For this review, take the finished solid that the model builds, in its own axes (mm). A direction names the side the tool comes from. Give positions to 0.01 mm unless a question says otherwise; leave off trailing zeros. Loops run counter-clockwise (first coordinate to the right, second up) from the corner with the lowest first, then second, coordinate; pieces in that order, holes last. Notation, with made-up numbers: (49, 3.25) - (94, 3.25) arc R24 ccw to (94, 33.25) - close; hole circle Ø5 at (39, 86.5). An arc over 180 degrees is marked (long way). Answer in a Markdown table with one row per item.
```python
from build123d import *

# Parameters (mm, degrees)
F0_W     = 160
F0_H     = 96
F0_W_2   = 143
F0_H_2   = 84
F0_R     = 1.5
F1_DEPTH = 10
F2_T     = -2


with BuildPart() as f1:
    # F0 (on Top) → F1 (new body)
    with BuildSketch(Plane.XY):
        Rectangle(F0_W, F0_H)
        Rectangle(F0_W_2, F0_H_2, mode=Mode.SUBTRACT)
        Rectangle(F0_W_2, F0_H_2)
        with Locations((-67.5, -38)):
            Circle(F0_R, mode=Mode.SUBTRACT)
        with Locations((67.5, -38)):
            Circle(F0_R, mode=Mode.SUBTRACT)
        with Locations((-67.5, 38)):
            Circle(F0_R, mode=Mode.SUBTRACT)
        with Locations((67.5, 38)):
            Circle(F0_R, mode=Mode.SUBTRACT)
    extrude(amount=F1_DEPTH)

    # F2
    f2_openings = [f1.faces().sort_by_distance(p)[0] for p in [
        (0, 0, 10),
    ]]
    offset(amount=F2_T, openings=f2_openings)


solid = f1.part
```
1. We need section D-D, the plane y = 15.5. Give the boundary of the cut face in (x, z).
Values:
| item | result |
|---|---|
| outline | (-80, 0) - (80, 0) - (80, 10) - (78, 10) - (78, 2) - (-78, 2) - (-78, 10) - (-80, 10) - close |
2. For faces 1 (the face through (68.886, -38.575, 4.93)), 2 (the face through (64.92, -35.635, 5.944)), list the 3-axis set-ups (+Z, -Z, +X, -X, +Y, -Y) from which the entire face can be reached by the end or side of a thin tool; tool diameter is ignored.
Values:
| item | result |
|---|---|
| face 1 | +Z, -Z |
| face 2 | +Z |
3. Wall thickness on line 1 (Y direction, x = 9, z = 7); line 2 (X direction, y = -34, z = 7.5); line 3 (Y direction, x = -67.5, z = 7.25): over which ranges is each line inside the solid? List them lowest first. Write a range as [from, to].
Values:
| item | result |
|---|---|
| line 1 | y = [-48, -46], [46, 48] |
| line 2 | x = [-80, -78], [78, 80] |
| line 3 | y = [-48, -46], [-41.5, -39.5], [-36.5, -34.5], [34.5, 36.5], [39.5, 41.5], [46, 48] |
4. We need section B-B, the plane x = -67.5. Give the boundary of the cut face in (y, z).
Values:
| item | result |
|---|---|
| outline | (-48, 0) - (-39.5, 0) - (-39.5, 10) - (-41.5, 10) - (-41.5, 2) - (-46, 2) - (-46, 10) - (-48, 10) - close; (-36.5, 0) - (36.5, 0) - (36.5, 10) - (34.5, 10) - (34.5, 2) - (-34.5, 2) - (-34.5, 10) - (-36.5, 10) - close; (39.5, 0) - (48, 0) - (48, 10) - (46, 10) - (46, 2) - (41.5, 2) - (41.5, 10) - (39.5, 10) - close |
5. We need section C-C, the plane y = -38. Give the boundary of the cut face in (x, z), and give its area (3 significant figures).
Values:
| item | result |
|---|---|
| outline | (-80, 0) - (-69, 0) - (-69, 10) - (-71, 10) - (-71, 2) - (-78, 2) - (-78, 10) - (-80, 10) - close; (-66, 0) - (66, 0) - (66, 10) - (64, 10) - (64, 2) - (-64, 2) - (-64, 10) - (-66, 10) - close; (69, 0) - (80, 0) - (80, 10) - (78, 10) - (78, 2) - (71, 2) - (71, 10) - (69, 10) - close |
| area | 404 mm^2 |
6. Mouldability with a two-part tool opening along Y and no side actions: class faces 3 (the face through (-70.08, 40.365, 5.944)), 4 (the face through (-1, -48, 5)), 5 (the face through (-68, -40, 10)) as released by +Y, released by -Y, zero draft, split by the parting line, or undercut.
Values:
| item | result |
|---|---|
| face 3 | undercut |
| face 4 | released by -Y |
| face 5 | zero draft |
7. Clearance check with a flat-ended pin moving along its axis: pin 1 (1.5 mm diameter, centred on x = -9.5, y = 1.5, fed in from +Z). State where the tip first meets the part, or that it passes through.
Values:
| item | result |
|---|---|
| pin 1 | stops at z = 2 |
8. We need section A-A, the plane z = 3.5. Count the separate pieces of the cut face and the enclosed holes in it, and give its area (3 significant figures).
Values:
| item | result |
|---|---|
| separate pieces | 5 |
| enclosed holes | 5 |
| area | 1,130 mm^2 |
